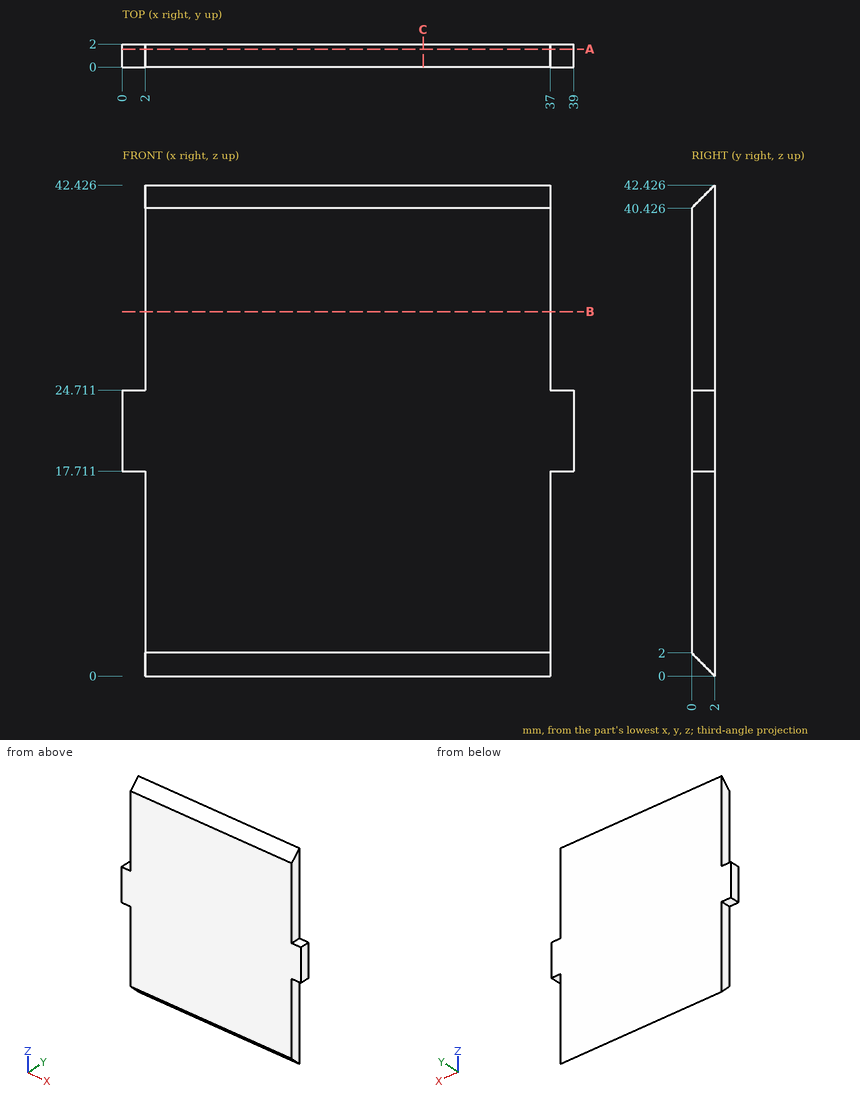
Here's the drawing with two shaded views (mm, measured from the low corner). I have some questions. Coordinates: 2 decimals unless noted, no trailing zeros. Order: outer loops, then holes, each group sorted by start corner. A loop starts at its lowest first (then second) coordinate and runs counter-clockwise, first axis right, second up.
Item 1: If we section it at A-A on y = 1.55: List the corners of the cut face in (x, z) for me, plus the area to 3 significant figures.
Result sheet:
outline: (0, 17.71) - (2, 17.71) - (2, 0.45) - (37, 0.45) - (37, 17.71) - (39, 17.71) - (39, 24.71) - (37, 24.71) - (37, 41.98) - (2, 41.98) - (2, 24.71) - (0, 24.71) - close
area: 1,480 mm2
Item 2: For P1, Ø1, axis at y = 1.5, z = 6, coming from the +X side; P2, Ø1, axis at y = 0.5, z = 6, coming from the -X side; P3, Ø0.6, axis at x = 38.5, y = 1, coming from the +Z side, each with a flat end and sliding along its axis, tell me the tip position at first contact or that it passes through.
Result sheet:
P1: stops at x = 37
P2: stops at x = 2
P3: stops at z = 24.71
Item 3: I need wall thicknesses on line 1 (X direction, y = 0.5, z = 16.5); line 2 (Z direction, x = 24, y = 0.3) (1 decimal); line 3 (Z direction, x = 34, y = 1.3) (1 decimal). Which ranges of each line are inside material? Lowest first, please.
Result sheet:
line 1: x = 2 to 37
line 2: z = 1.7 to 40.7
line 3: z = 0.7 to 41.7
Item 4: If we section it at B-B on z = 31.5: List the corners of the cut face in (x, y) for me.
Result sheet:
outline: (2, 0) - (37, 0) - (37, 2) - (2, 2) - close
Item 5: If we section it at C-C on x = 26: List the corners of the cut face in (y, z) for me.
Result sheet:
outline: (0, 2) - (2, 0) - (2, 42.43) - (0, 40.43) - close
